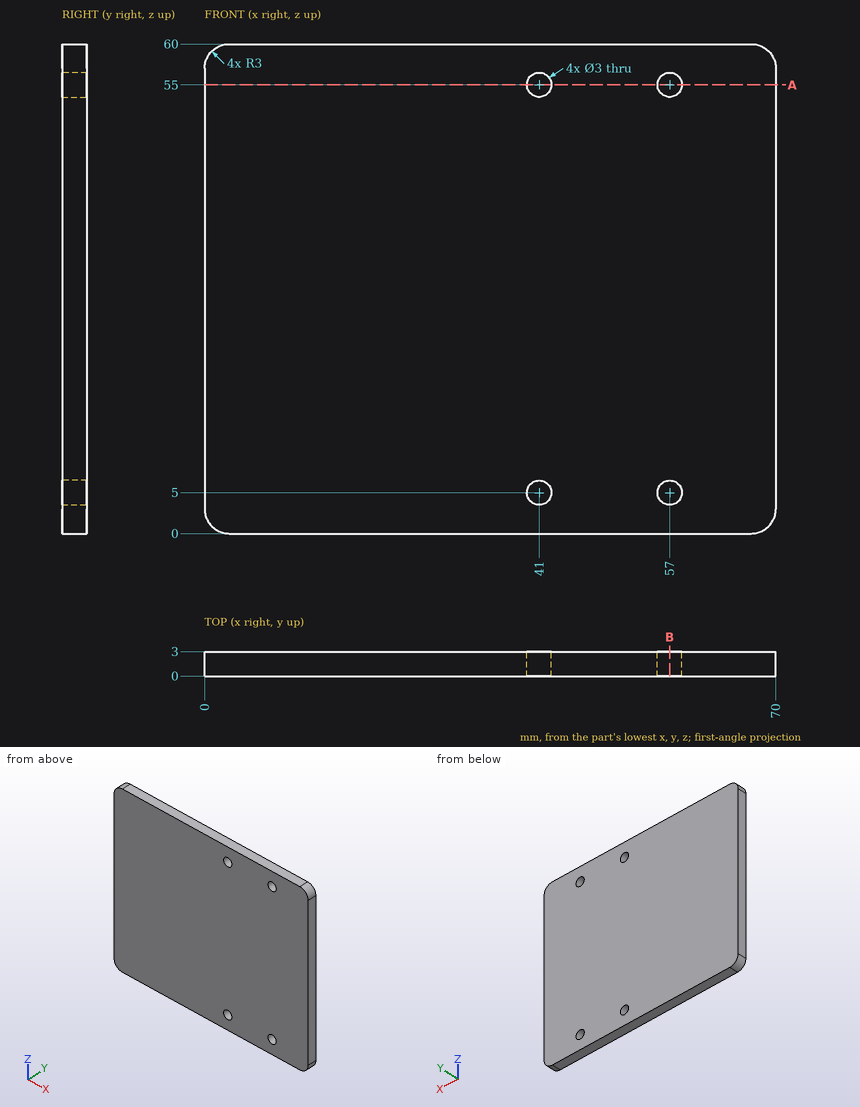
Can you work these out from the drawing? Everything is in mm from the part's minimum corner. Round coordinates to 2 decimals unless told otherwise and drop trailing zeros. Loops run counter-clockwise (first coordinate to the right, second up) from the corner with the lowest first, then second, coordinate; pieces in that order, holes last. Notation, with made-up numbers: (66, -31) -> (118, -31) arc R17 cw to (118, -11) -> close; hole circle Ø9 at (22, 89). An arc over 180 degrees is marked (long way). Answer in a Markdown table with one row per item.
Item 1: If I drill on probe 1 along X at (y, z) = (2.1, 5); probe 2 along Z at (x, y) = (42, 1.7); probe 3 along X at (y, z) = (0.2, 6), over which ranges is the centre line in solid material (lowest first)?
Answer block:
| item | result |
|---|---|
| probe 1 | 0 to 39.5, 42.5 to 55.5, 58.5 to 70 |
| probe 2 | 0 to 3.88, 6.12 to 53.88, 56.12 to 60 |
| probe 3 | 0 to 39.88, 42.12 to 55.88, 58.12 to 70 |
Item 2: Suppose I cut it at B-B, the plane x = 57. List the corners of the cut face in (y, z) for me, plus the area to 3 significant figures.
Answer block:
| item | result |
|---|---|
| outline | (0, 0) -> (3, 0) -> (3, 3.5) -> (0, 3.5) -> close; (0, 6.5) -> (3, 6.5) -> (3, 53.5) -> (0, 53.5) -> close; (0, 56.5) -> (3, 56.5) -> (3, 60) -> (0, 60) -> close |
| area | 162 mm² |
Item 3: Suppose I cut it at A-A, the plane z = 55. List the corners of the cut face in (x, y) for me, plus the area to 3 significant figures.
Answer block:
| item | result |
|---|---|
| outline | (0, 0) -> (39.5, 0) -> (39.5, 3) -> (0, 3) -> close; (42.5, 0) -> (55.5, 0) -> (55.5, 3) -> (42.5, 3) -> close; (58.5, 0) -> (70, 0) -> (70, 3) -> (58.5, 3) -> close |
| area | 192 mm² |
Item 4: Will these pins go through, and if not, where does the flat tip stop? P1, Ø2.5, axis at x = 57, z = 55, coming from the -Y side; P2, Ø3.5, axis at x = 41, z = 5, coming from the +Y side.
Answer block:
| item | result |
|---|---|
| P1 | through |
| P2 | y = 3 |
